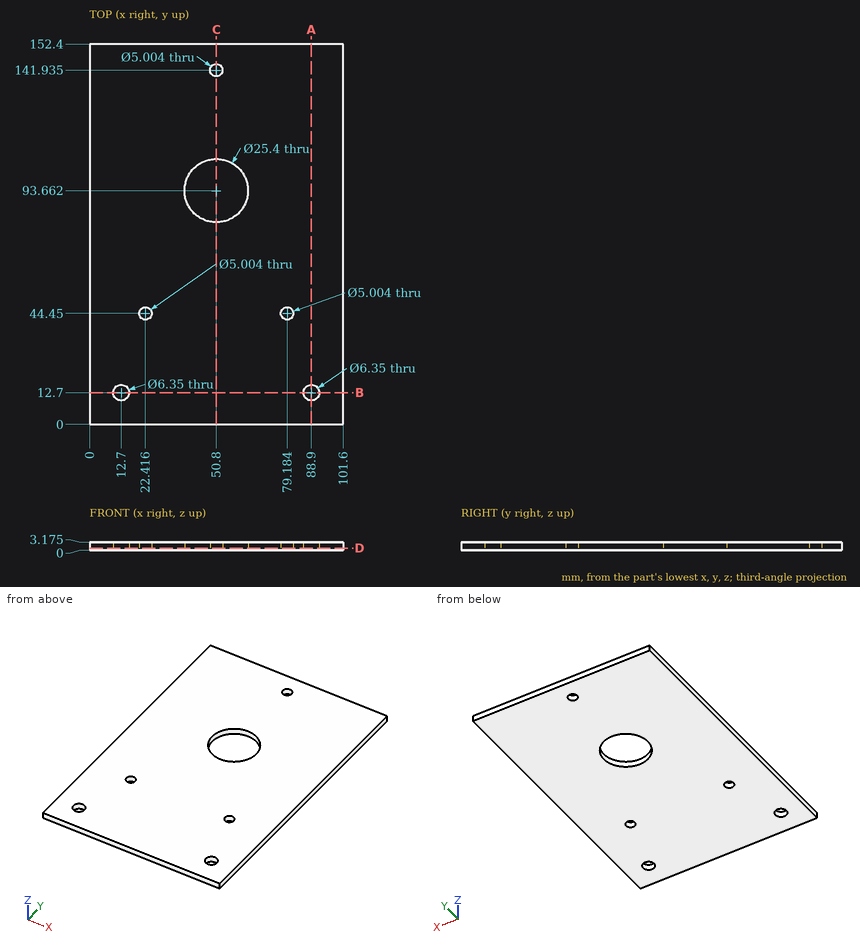
For this review, use the dimensioned drawing (mm, ordinates from the lowest corner) and the shaded views. Round coordinates to 2 decimals unless told otherwise and drop trailing zeros. Order: outer loops, then holes, each group sorted by start corner. A loop starts at its lowest first (then second) coordinate and runs counter-clockwise, first axis right, second up. Notation, with made-up numbers: M 21,-7 L 27,-7 A20 cw 27,-3 Z; hole C -23.5,88 d8. An arc over 180 degrees is marked long. Write each question's results on one line, items separated by ' | '. Start each with the question number.
1. Add section C-C (x = 50.8). State the section outline as (y, z) points (1 decimal).
2. Add section D-D (z = 0.9). State how many separate pieces and enclosed holes the cut face has, then the cut area to 3 significant figures.
3. Add section A-A (x = 88.9). State the section outline as (y, z) points (1 decimal).
4. To check wall thickness, follow L1, parallel to X at y = 12.7, z = 1.3 (1 decimal); L2, parallel to X at y = 44.45, z = 2; L3, parallel to Y at x = 15, z = 0.5. State the ranges of each line that lie inside material, in increasing order. Write a range as [from, to].
5. Add section B-B (y = 12.7). State the section outline as (x, z) points (1 decimal).
Output values:
1) outline: M 0,0 L 81,0 L 81,3.2 L 0,3.2 Z; M 106.4,0 L 139.4,0 L 139.4,3.2 L 106.4,3.2 Z; M 144.4,0 L 152.4,0 L 152.4,3.2 L 144.4,3.2 Z
2) separate pieces: 1 | enclosed holes: 6 | area: 14,900 mm^2
3) outline: M 0,0 L 9.5,0 L 9.5,3.2 L 0,3.2 Z; M 15.9,0 L 152.4,0 L 152.4,3.2 L 15.9,3.2 Z
4) L1: [0, 9.5], [15.9, 85.7], [92.1, 101.6] | L2: [0, 19.91], [24.92, 76.68], [81.69, 101.6] | L3: [0, 10.51], [14.89, 152.4]
5) outline: M 0,0 L 9.5,0 L 9.5,3.2 L 0,3.2 Z; M 15.9,0 L 85.7,0 L 85.7,3.2 L 15.9,3.2 Z; M 92.1,0 L 101.6,0 L 101.6,3.2 L 92.1,3.2 Z
